Input: dimensioned drawing with shaded views. Units: mm. Origin: part minimum x, y, z. Give positions to 0.01 mm unless a question says otherwise; leave off trailing zeros. Loops run counter-clockwise (first coordinate to the right, second up) from the corner with the lowest first, then second, coordinate; pieces in that order, holes last. Notation, with made-up numbers: (0, -20.75) -> (42, -20.75) arc R19 ccw to (42, 2.25) -> close; hole circle Ø6 at (72.25, 8.5). An arc over 180 degrees is marked (long way). Answer as a JSON object with one key per item and string values.
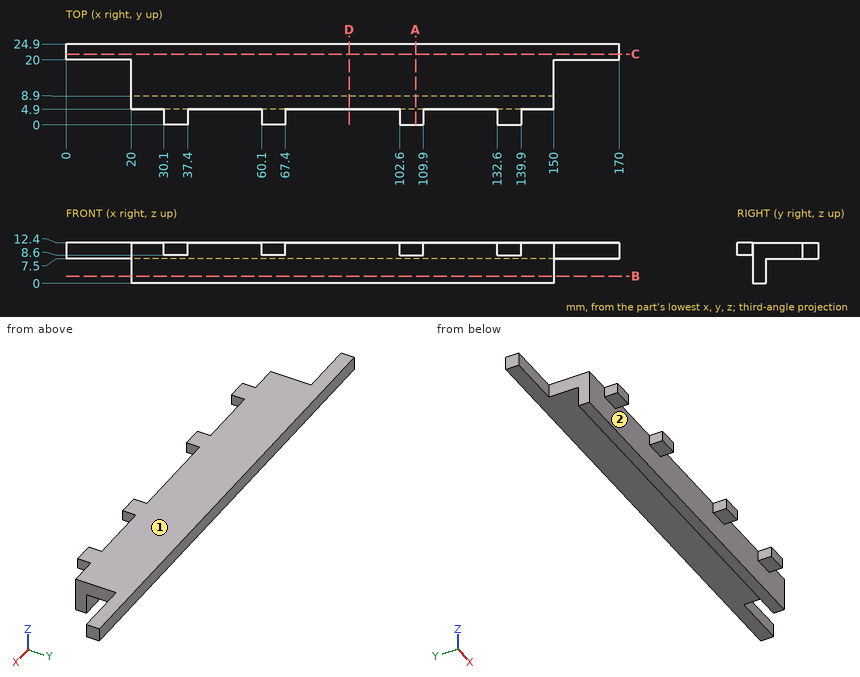
Q1. Section A-A, the plane x = 107.5. Return the cut outline in (y, z), then the cut area to 3 significant figures.
Evaluation:
{"outline": "(0, 8.6) -> (4.9, 8.6) -> (4.9, 0) -> (8.9, 0) -> (8.9, 7.5) -> (24.9, 7.5) -> (24.9, 12.4) -> (0, 12.4) -> close", "area": "147 mm2"}
Q2. Section C-C, the plane y = 21.75. Return the cut outline in (x, z).
Evaluation:
{"outline": "(0, 7.5) -> (170, 7.5) -> (170, 12.4) -> (0, 12.4) -> close"}
Q3. Section B-B, the plane z = 2.25. Return the cut outline in (x, y), then the cut area to 3 significant figures.
Evaluation:
{"outline": "(20, 4.9) -> (150, 4.9) -> (150, 8.9) -> (20, 8.9) -> close", "area": "520 mm2"}
Q4. Section D-D, the plane x = 87. Return the cut outline in (y, z), then the cut area to 3 significant figures.
Evaluation:
{"outline": "(4.9, 0) -> (8.9, 0) -> (8.9, 7.5) -> (24.9, 7.5) -> (24.9, 12.4) -> (4.9, 12.4) -> close", "area": "128 mm2"}
Q5. Ray query, line 1 along Y through (x, z) = (9.5, 10.75); line 2 along Y through (x, z) = (70, 9.5); line 3 along Z through (x, y) = (23, 16.5). Return the intervals inside material, ascending.
Evaluation:
{"line 1": "y = 20 to 24.9", "line 2": "y = 4.9 to 24.9", "line 3": "z = 7.5 to 12.4"}
Q6. Pin query (flat end, axial travel): pin 1 (1.9 mm diameter, centred on y = 2.5, z = 10, fed in from +X); pin 2 (2.5 mm diameter, centred on x = 159.5, z = 11, fed in from -Y); pin 3 (3 mm diameter, centred on x = 139.5, y = 12, fed in from -Z); pin 4 (8 mm diameter, centred on x = 115.5, y = 9.5, fed in from -Z). Return the tip coordinate at first contact, or that it passes through.
Evaluation:
{"pin 1": "stops at x = 139.9", "pin 2": "stops at y = 20", "pin 3": "stops at z = 7.5", "pin 4": "stops at z = 0"}
Q7. Draft query along X for the marked faces 1 and 2. Return one class per face: +X half, -X half, draft (parallel to the pull), parting line (faces both ways), or undercut.
Evaluation:
{"face 1": "draft", "face 2": "undercut"}
